Autodesk Inventor part; units mm, degrees
ref_plane "YZ Plane" through (0, 0, 0) normal (1, 0, 0) x (0, 1, 0)
ref_plane "XZ Plane" through (0, 0, 0) normal (0, 1, 0) x (-1, 0, 0)
ref_plane "XY Plane" through (0, 0, 0) normal (0, 0, 1) x (1, 0, 0)
sketch "Sketch1" plane through (0, 0, 0) normal (0, 1, 0) x (-1, 0, 0)
  circle A0 centre (0, 0) radius 6.35
  dimension "d0" = 12.7
extrude "Extrusion1" add sketch "Sketch1" along normal blind 12.7
sketch "Sketch2" plane through (0, 0, 0) normal (0, -1, 0) x (1, 0, 0)
  circle A0 centre (0, 0) radius 6.985
  dimension "d3" = 13.97
extrude "Extrusion2" add sketch "Sketch2" along normal blind 1.27
sketch "Sketch3" plane through (0, -1.27, 0) normal (0, -1, 0) x (1, 0, 0)
  circle A0 centre (0, 0) radius 6.35
  dimension "d6" = 12.7
extrude "Extrusion3" add sketch "Sketch3" along normal blind 28.575
sketch "Sketch4" plane through (0, 0, 0) normal (0, 0, 1) x (1, 0, 0)
  line L0 (-6.35, -29.845) -> (6.35, -29.845)
  line L1 (-6.35, -29.845) -> (-6.35, -1.27)
  line L2 (-6.985, -1.27) -> (6.985, -1.27)
  line L3 (-6.35, -1.27) -> (-6.35, -29.845)
  circle A0 centre (18.9357, -27.94) radius 25.4
  circle A1 centre (18.9357, -27.94) radius 22.86
  line L4 (-6.3928, -29.845) -> (44.2642, -29.845)
  point P0 (0, 0)
  point P1 (0, -1.27)
  point P2 (41.7162, -29.845)
  point P3 (-3.8448, -29.845)
  point P4 (-6.35, -25.5331)
  dimension "d11" = 45.72
  dimension "d12" = 26.67
  dimension "d13" = 50.8
  dimension "d14" = 25.2857
extrude "Extrusion4" add sketch "Sketch4" along normal mid plane 15.24 contours L1 A0 L4 A1 L0
sketch "Sketch5" plane through (-6.35, -29.845, 7.62) normal (-1, 0, 0) x (0, 0, 1)
  line L0 (-2.54, 4.318) -> (-2.54, 0)
  line L1 (-2.54, 0) -> (-12.7, 0)
  line L2 (-12.7, 0) -> (-12.7, 4.318)
  line L3 (0, 4.3119) -> (0, 0)
  line L4 (-15.24, 0) -> (-15.24, 4.3119)
  line L5 (-7.62, 4.3119) -> (0, 4.3119)
  line L6 (-12.7, 4.3119) -> (-2.54, 4.3119)
  point P0 (-7.62, 29.845)
  point P1 (-2.5663, 0)
  point P2 (-3.81, 4.3119)
  point P3 (-2.54, 4.3119)
  dimension "d17" = 2.54
  dimension "d18" = 2.54
  dimension "d21" = 4.3119
  dimension "d22" = 0.0061
  dimension "d23" = 0.0061
extrude "Extrusion5" add sketch "Sketch5" against normal blind 50.165
sketch "Sketch6" plane through (0, 0, 0) normal (0, 0, 1) x (1, 0, 0)
  arc A0 (41.7162, -29.845) -> (-3.8448, -29.845) centre (18.9357, -27.94) ccw
  circle A1 centre (18.9357, -27.94) radius 1.905
  point P0 (0, 0)
  point P1 (4.5348, -10.1863)
  point P2 (0, -15.133)
  dimension "d26" = 3.81
extrude "Extrusion6" add sketch "Sketch6" along normal mid plane 25.4
properties part number "Wheel sheild (H)"
Can you work these out from the model? Positions are in its coordinate system, mm. A direction names the side the tool comes from. Coordinates: 2 decimals unless noted, no trailing zeros. Loops run counter-clockwise (first coordinate to the right, second up) from the corner with the lowest first, then second, coordinate; pieces in that order, holes last.
Item 1: I'm going to push flat-ended pins straight in: pin 1 (8 mm diameter, centred on x = 22, y = -22.5, fed in from +Z); pin 2 (8 mm diameter, centred on x = 19, z = -2, fed in from +Y); pin 3 (10 mm diameter, centred on y = 5.5, z = -6, fed in from -X). Where does each tip first touch, or does it pass through?
Answers below:
pin 1: stops at z = 5.08
pin 2: stops at y = -2.54
pin 3: stops at x = -6.27
Item 2: Suppose I cut it at B-B (x = 32). Please give me the cut outline in (y, z) (3 decimals), then the cut area to 3 significant figures.
Answers below:
outline: (-29.845, -5.08) - (-25.533, -5.08) - (-25.533, 5.08) - (-29.845, 5.08) - close; (-9.181, -7.62) - (-6.157, -7.62) - (-6.157, 7.62) - (-9.181, 7.62) - close
area: 89.9 mm2
Item 3: Please list where these lines run through material, in increasing order: L1, parallel to X at y = -7, z = 5.75; L2, parallel to X at y = -27.94, z = 0.25; L3, parallel to X at y = -19, z = 3.75.
Answers below:
L1: x = -2.69 to 2.69, 4.56 to 9.77, 28.11 to 33.31
L2: x = -6.35 to 44.34
L3: x = -5.12 to 5.12, 39.98 to 42.71
Item 4: Suppose I cut it at D-D (x = -3). Please give me the cut outline in (y, z) (3 decimals), then the cut area to 3 significant figures.
Answers below:
outline: (-29.845, -5.597) - (-21.505, -5.597) - (-21.505, -7.62) - (-15.134, -7.62) - (-15.134, -5.597) - (-1.27, -5.597) - (-1.27, -6.308) - (0, -6.308) - (0, -5.597) - (12.7, -5.597) - (12.7, 5.597) - (0, 5.597) - (0, 6.308) - (-1.27, 6.308) - (-1.27, 5.597) - (-15.134, 5.597) - (-15.134, 7.62) - (-21.505, 7.62) - (-21.505, 5.597) - (-29.845, 5.597) - close
area: 504 mm2
Item 5: Suppose I cut it at C-C (z = 1.75). Please give me the cut outline in (x, y) (3 decimals).
Answers below:
outline: (-6.762, -1.27) - (-6.104, -1.27) - (-6.104, -23.678) arc R25.4 ccw to (-6.35, -25.533) - (-6.35, -29.845) - (44.264, -29.845) arc R25.4 ccw to (6.104, -6.019) - (6.104, -1.27) - (6.762, -1.27) - (6.762, 0) - (6.104, 0) - (6.104, 12.7) - (-6.104, 12.7) - (-6.104, 0) - (-6.762, 0) - close; hole (6.104, -25.533) - (41.669, -25.533) arc R22.86 ccw to (6.104, -9.021) - close
Item 6: Suppose I cut it at A-A (y = -24.5). Please give me the cut outline in (x, z).
Answers below:
outline: (-6.23, -7.62) - (-3.66, -7.62) - (-3.66, -5.19) arc R6.35 ccw (long way) to (-3.66, 5.19) - (-3.66, 7.62) - (-6.23, 7.62) - (-6.23, 1.23) arc R6.35 ccw to (-6.23, -1.23) - close; (41.54, -7.62) - (44.1, -7.62) - (44.1, 7.62) - (41.54, 7.62) - close
Item 7: If we mould it in two halves opening along X, with no side actions, what happens to faces 1 (the face through (19, -29.845, 0)), 2 (the face through (-0.909, -0.626, -6.926)), 3 (the face through (19.815, -29.63, -8.837))? For each: released by +X, released by -X, zero draft, split by the parting line, or undercut.
Answers below:
face 1: zero draft
face 2: split by the parting line
face 3: undercut
Item 8: Which directions (+Z, -Z, +X, -X, +Y, -Y) give clear straight access to the entire face, cutting with the end or side of a thin tool? Please do faces 4 (the face through (6.347, -19.203, 0.197)), 5 (the face through (1.38, 6.26, 6.2)), 6 (the face through (18.69, -29.83, 8.84)).
Answers below:
face 4: none
face 5: +Y
face 6: +Z
